Autodesk Inventor part; units mm, degrees
ref_plane "YZ Plane" through (0, 0, 0) normal (1, 0, 0) x (0, 1, 0)
ref_plane "XZ Plane" through (0, 0, 0) normal (0, 1, 0) x (-1, 0, 0)
ref_plane "XY Plane" through (0, 0, 0) normal (0, 0, 1) x (1, 0, 0)
sketch "Sketch1" plane through (0, 0, 0) normal (0, 1, 0) x (-1, 0, 0)
  line L0 (0, 0) -> (215.9, 0)
  line L1 (215.9, 0) -> (215.9, -25.4)
  line L2 (215.9, -25.4) -> (0, -25.4)
  line L3 (0, -25.4) -> (0, 0)
  dimension "d0" = 215.9
  dimension "d1" = 25.4
extrude "Extrusion1" add sketch "Sketch1" along normal blind 2.54
sketch "Sketch2" plane through (0, 2.54, 0) normal (0, 1, 0) x (1, 0, 0)
  line L0 (0, 0) -> (0, 25.4)
  line L1 (0, 25.4) -> (-215.9, 25.4)
  line L2 (0, 0) -> (-2.54, 0)
  line L3 (-2.54, 2.54) -> (-2.54, 25.4)
  line L4 (-2.54, 25.4) -> (0, 25.4)
  line L5 (0, 25.4) -> (0, 0)
  line L6 (-215.9, 25.4) -> (-215.9, 0)
  line L7 (0, 0) -> (-215.9, 0)
  line L8 (-215.9, 0) -> (-215.9, 2.54)
  line L9 (-213.36, 2.54) -> (-2.54, 2.54)
  line L10 (0, 2.54) -> (0, 0)
  line L11 (-215.9, 0) -> (0, 0)
  line L12 (-215.9, 0) -> (-213.36, 0)
  line L13 (-213.36, 2.54) -> (-213.36, 25.4)
  line L14 (-213.36, 25.4) -> (-215.9, 25.4)
  line L15 (-215.9, 25.4) -> (-215.9, 0)
  dimension "d4" = 2.54
  dimension "d5" = 2.54
  dimension "d6" = 2.54
extrude "Extrusion2" add sketch "Sketch2" along normal blind 25.4 contours L2 L7 L6 L1 L13 L9 L3 L0
properties part number "batterymount" material "UHMW, Black"
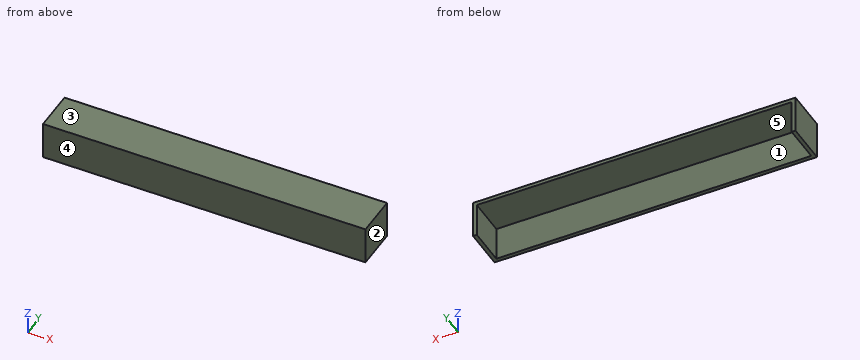
Source: CAD feature listing. Evaluate the final solid. Frame: model axes, mm. Face numbers are marked on the shaded views. A direction names the side the tool comes from. Give positions to 0.01 mm unless a question says otherwise; leave off trailing zeros. Order: outer loops, then holes, each group sorted by start corner. A loop starts at its lowest first (then second) coordinate and runs counter-clockwise, first axis right, second up. Notation, with made-up numbers: (56, 35) -> (101, 35) arc R11 cw to (101, 48) -> close; hole circle Ø5 at (-23.5, 63.25). An arc over 180 degrees is marked (long way). Write item = value, one per line.
Item 1: Mould query, pull axis X, two halves, no side actions, for the marked faces 1, 2 and 3. Classes: +X half, -X half, draft (parallel to the pull), parting line (faces both ways), or undercut.
Check result:
face_1 = undercut
face_2 = +X half
face_3 = draft
Item 2: Contact query for flat-ended pins moving along their axis: pin 1 (1 mm diameter, centred on x = -63, z = -22.5, fed in from +Y); pin 2 (1 mm diameter, centred on x = -187.5, y = 6.5, fed in from -Z). Output: stop coordinate, or through.
Check result:
pin_1 = 2.54
pin_2 = -2.54
Item 3: Section query A-A (y = 19.75). Output: boundary loops of the cut face in (x, z).
Check result:
outline = (-215.9, -25.4) -> (-213.36, -25.4) -> (-213.36, -2.54) -> (-2.54, -2.54) -> (-2.54, -25.4) -> (0, -25.4) -> (0, 0) -> (-215.9, 0) -> close
Item 4: Set-up query: the marked faces 4 and 5. Return all of +Z, -Z, +X, -X, +Y, -Y with unobstructed straight access to the full face (end or side cutting, diameter ignored); none if empty.
Check result:
face_4 = +Z, -Z, +X, -X, -Y
face_5 = -Z, +Y
Item 5: Ray query, probe 1 along X at (y, z) = (5, -18.5); probe 2 along Z at (x, y) = (-182, 11.75); probe 3 along Y at (x, z) = (-77, -21.25). Return the intervals inside material, ascending.
Check result:
probe_1 = -215.9 to -213.36, -2.54 to 0
probe_2 = -2.54 to 0
probe_3 = 0 to 2.54
Item 6: Section query C-C (x = -92). Output: boundary loops of the cut face in (y, z).
Check result:
outline = (0, -25.4) -> (2.54, -25.4) -> (2.54, -2.54) -> (27.94, -2.54) -> (27.94, 0) -> (0, 0) -> close
Item 7: Section query B-B (z = -15.75). Output: boundary loops of the cut face in (x, y), then the cut area to 3 significant figures.
Check result:
outline = (-215.9, 0) -> (0, 0) -> (0, 27.94) -> (-2.54, 27.94) -> (-2.54, 2.54) -> (-213.36, 2.54) -> (-213.36, 27.94) -> (-215.9, 27.94) -> close
area = 677 mm²
